```python
from build123d import *

# Parameters (mm, degrees)
F0_R           = 203.2
F1_DEPTH       = 19.05
F2_R           = 144.399
F2_R_2         = 131.699
F3_DEPTH       = 6.35
F4_R           = 3.175
F6_D           = 22.225
F8_D           = 14
F8_CBORE_D     = 24
F8_CBORE_DEPTH = 7.5
F9_W           = 12.7
F9_H           = 38.1
F10_DEPTH      = 45.72
F12_D          = 5.1054
F12_DEPTH      = 15.875
F12_TIP        = 1.5338169022
F14_D          = 8.73125


# Not quite as in the source:
# - a length typed as a fraction of an inch, garbled in the dataset ("3 / 203.2 mm" for 3/8 in), is restored


with BuildPart() as f1:
    # F0 (on Right) → F1 (new body)
    with BuildSketch(Plane.YZ):
        Circle(F0_R)
    extrude(amount=-F1_DEPTH)

    # F2 (on face) → F3 (join)
    with BuildSketch(Plane.YZ):
        Circle(F2_R)
        Circle(F2_R_2, mode=Mode.SUBTRACT)
    extrude(amount=F3_DEPTH)

    # F4
    f4_edges = [f1.edges().sort_by_distance(p)[0] for p in [
        (0, -131.699, 0),
    ]]
    fillet(f4_edges, radius=F4_R)

    # F6 (through all)
    with Locations(Plane(origin=(-19.05, 0, 0), x_dir=(0, -1, 0), z_dir=(-1, 0, 0))):
        with Locations((0, 177.8), (153.9793167929, 88.9), (-153.9793167929, 88.9), (-153.9793167929, -88.9), (153.9793167929, -88.9), (0, -177.8)):
            Hole(F6_D / 2)

    # F8 (through all)
    with Locations(Plane(origin=(-19.05, 0, 0), x_dir=(0, -1, 0), z_dir=(-1, 0, 0))):
        with Locations((0, 0)):
            CounterBoreHole(F8_D / 2, F8_CBORE_D / 2, F8_CBORE_DEPTH)

    # F9 (on face) → F10 (join)
    with BuildSketch(Plane(origin=(-19.05, 0, 0), x_dir=(0, -1, 0), z_dir=(-1, 0, 0))):
        with Locations((38.1, 0)):
            Rectangle(F9_W, F9_H)
        with Locations((-38.1, 0)):
            Rectangle(F9_W, F9_H)
    extrude(amount=F10_DEPTH)

    # F12
    with Locations(Plane(origin=(-64.77, 0, 0), x_dir=(0, -1, 0), z_dir=(-1, 0, 0))):
        with Locations((-38.1, 12.7), (-38.1, -12.7), (38.1, 12.7), (38.1, -12.7)):
            Hole(F12_D / 2, depth=F12_DEPTH)
            with Locations((0, 0, -(F12_DEPTH + F12_TIP / 2))):  # 118° drill point
                Cone(0, F12_D / 2, F12_TIP, mode=Mode.SUBTRACT)

    # F14 (through all)
    with Locations(Plane(origin=(-19.05, 0, 0), x_dir=(0, -1, 0), z_dir=(-1, 0, 0))):
        with Locations((0, 120.65)):
            Hole(F14_D / 2)


solid = f1.part
```
The listing builds one solid part. Answer for the finished solid, in the listing's coordinates (mm). A direction names the side the tool comes from. Coordinates: 2 decimals unless noted, no trailing zeros. Loops run counter-clockwise (first coordinate to the right, second up) from the corner with the lowest first, then second, coordinate; pieces in that order, holes last. Notation, with made-up numbers: (21, 70) - (41, 70) arc R11 cw to (41, 90) - close; hole circle Ø8 at (5, -16). An arc over 180 degrees is marked (long way). Write item = value, one per line.
1) Find the intervals of material crossed by line 1 along Z through (x, y) = (-16, 0); line 2 along Z through (x, y) = (-56.75, -38.1); line 3 along Y through (x, z) = (-55, 12.7), in increasing order.
Responses:
line_1 = -203.2 to -188.91, -166.69 to -12, 12 to 116.28, 125.02 to 166.69, 188.91 to 203.2
line_2 = -19.05 to -15.25, -10.15 to 10.15, 15.25 to 19.05
line_3 = -44.45 to -40.65, -35.55 to -31.75, 31.75 to 35.55, 40.65 to 44.45
2) Each of these flat-tipped pins is pushed along its axis until it touches: P1, Ø6.5, axis at x = -34.5, y = 39.5, coming from the -Z side; P2, Ø4, axis at x = -36, y = -41, coming from the +Z side; P3, Ø1.5, axis at x = -31, z = -8.5, coming from the -Y side; P4, Ø10, axis at y = -18.5, z = 126, coming from the +X side. Where does it stop, or does it pass through?
Responses:
P1 = -19.05
P2 = 19.05
P3 = -44.45
P4 = 6.35
3) Section C-C (z = -88.9) is taken. Count the separate pieces of the cut face and the enclosed holes in it, plus the area to 3 significant figures.
Responses:
separate_pieces = 3
enclosed_holes = 0
area = 6,330 mm^2
4) Section A-A (x = -58.5) is taken. Determine the outline of the cut face in (y, z).
Responses:
outline = (-44.45, -19.05) - (-31.75, -19.05) - (-31.75, 19.05) - (-44.45, 19.05) - close; (31.75, -19.05) - (44.45, -19.05) - (44.45, 19.05) - (31.75, 19.05) - close; hole circle Ø5.11 at (-38.1, -12.7); hole circle Ø5.11 at (-38.1, 12.7); hole circle Ø5.11 at (38.1, -12.7); hole circle Ø5.11 at (38.1, 12.7)
5) Section D-D (z = 177.8) is taken. Determine the outline of the cut face in (x, y).
Responses:
outline = (-19.05, -98.37) - (0, -98.37) - (0, -11.11) - (-19.05, -11.11) - close; (-19.05, 11.11) - (0, 11.11) - (0, 98.37) - (-19.05, 98.37) - close
6) Determine the mould class of faces 6 (the face through (-9.392, -1.447, -166.782)), 7 (the face through (-42, 38, -19.05)), 8 (the face through (-9.392, -44.05, -198.368)) for opening direction Y: pulls with the +Y half, pulls with the -Y half, needs draft (parallel to the pull), parting line crosses it, or undercut.
Responses:
face_6 = undercut
face_7 = needs draft
face_8 = parting line crosses it
7) Which of the six approach directions +Z, -Z, +X, -X, +Y, -Y give full straight-line access (tool end or side, diameter ignored) to faces 1 (the face through (-11.55, -5.2, -5.2)), 2 (the face through (0, -138.3, -42.3)), 3 (the face through (-42, 38, 19.05)), 4 (the face through (-42, 44.45, 0)), 5 (the face through (-42, 31.75, 0))?
Responses:
face_1 = -X
face_2 = +X
face_3 = +Z, -X, +Y, -Y
face_4 = +Z, -Z, -X, +Y
face_5 = +Z, -Z, -X
